Work out the finished part from the listing and answer in its coordinate system (mm). Round coordinates to 2 decimals unless told otherwise and drop trailing zeros. Order: outer loops, then holes, each group sorted by start corner. A loop starts at its lowest first (then second) coordinate and runs counter-clockwise, first axis right, second up. Notation, with made-up numbers: (39.5, 37) -> (45.5, 37) arc R24 ccw to (45.5, 71) -> close; hole circle Ø7 at (58, 72). An arc over 180 degrees is marked (long way). Use one line per item in the form item = value.
```python
from build123d import *

# Parameters (mm, degrees)
SKETCH_1_W          = 15
SKETCH_1_H          = 15
SKETCH_1_W_2        = 12
SKETCH_1_H_2        = 12
EXTRUDE_1_DEPTH     = 200
SKETCH_2_R          = 1.6
CUT_EXTRUDE_1_DEPTH = 201.701893364
SKETCH_3_R          = 1.6
CUT_EXTRUDE_2_DEPTH = 201.701893364


with BuildPart() as part:
    # ｽｹｯﾁ1 → ﾎﾞｽ - 押し出し1 (new body)
    with BuildSketch(Plane(origin=(0, 0, 0), x_dir=(1, 0, 0), z_dir=(0, 1, 0))):
        Rectangle(SKETCH_1_W, SKETCH_1_H)
        Rectangle(SKETCH_1_W_2, SKETCH_1_H_2, mode=Mode.SUBTRACT)
    extrude(amount=EXTRUDE_1_DEPTH)

    # ｽｹｯﾁ2 → ｶｯﾄ - 押し出し1 (cut, through all)
    with BuildSketch(Plane.XY.offset(7.5)):
        with Locations((0, 192.5)):
            Circle(SKETCH_2_R)
        with Locations((0, 7.5)):
            Circle(SKETCH_2_R)
    extrude(amount=-CUT_EXTRUDE_1_DEPTH, mode=Mode.SUBTRACT)

    # ｽｹｯﾁ3 → ｶｯﾄ - 押し出し2 (cut, through all)
    with BuildSketch(Plane(origin=(7.5, 0, 0), x_dir=(0, 0, -1), z_dir=(1, 0, 0))):
        with Locations((0, 177.5)):
            Circle(SKETCH_3_R)
        with Locations((0, 22.5)):
            Circle(SKETCH_3_R)
        with Locations((0, 37.5)):
            Circle(SKETCH_3_R)
    extrude(amount=-CUT_EXTRUDE_2_DEPTH, mode=Mode.SUBTRACT)


solid = part.part
```
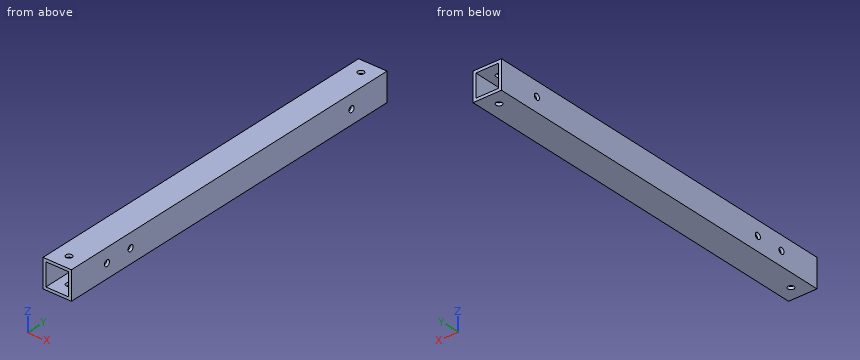
Item 1: The part is cut by section A-A, the plane y = 154.5. Give the vertices of the cut face in (x, z).
Findings:
outline = (-7.5, -7.5) -> (7.5, -7.5) -> (7.5, 7.5) -> (-7.5, 7.5) -> close; hole (-6, -6) -> (6, -6) -> (6, 6) -> (-6, 6) -> close
Item 2: The part is cut by section B-B, the plane x = -3.25. Give the vertices of the cut face in (y, z).
Findings:
outline = (0, -7.5) -> (200, -7.5) -> (200, -6) -> (0, -6) -> close; (0, 6) -> (200, 6) -> (200, 7.5) -> (0, 7.5) -> close
Item 3: A flat-ended cylindrical pin translates along its axis: P1, Ø2.5, axis at y = 22.5, z = 0, coming from the +X side. Find the tip coordinate at first contact, or state that the pin passes through.
Findings:
P1 = through
Item 4: Consider line 1 along Y through (x, z) = (0, -6.4); line 2 along Y through (x, z) = (-6.6, 0); line 3 along X through (y, z) = (175, -3.5). Determine where each line is inside the solid, lowest interval first.
Findings:
line_1 = 0 to 5.9, 9.1 to 190.9, 194.1 to 200
line_2 = 0 to 20.9, 24.1 to 35.9, 39.1 to 175.9, 179.1 to 200
line_3 = -7.5 to -6, 6 to 7.5
